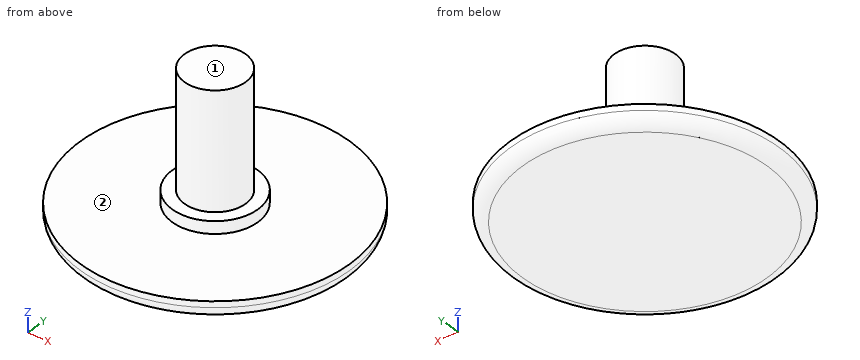
from build123d import *

# Parameters (mm, degrees)
F0_R     = 11
F1_DEPTH = 1.5
F2_R     = 3.5
F3_DEPTH = 1
F4_R     = 2.5
F5_DEPTH = 9.5
F6_R     = 1


with BuildPart() as f1:
    # F0 (on Top) → F1 (new body)
    with BuildSketch(Plane.XY):
        Circle(F0_R)
    extrude(amount=-F1_DEPTH)

    # F2 (on face) → F3 (join)
    with BuildSketch(Plane.XY):
        Circle(F2_R)
    extrude(amount=F3_DEPTH)

    # F4 (on face) → F5 (join)
    with BuildSketch(Plane.XY.offset(1)):
        Circle(F4_R)
    extrude(amount=F5_DEPTH)

    # F6
    f6_edges = [f1.edges().sort_by_distance(p)[0] for p in [
        (-11, 0, -1.5),
    ]]
    fillet(f6_edges, radius=F6_R)


solid = f1.part
Geometry: final body of the model. Coordinates: model frame, mm. Face numbers are marked on the shaded views. A direction names the side the tool comes from. Give positions to 0.01 mm unless a question says otherwise; leave off trailing zeros. Order: outer loops, then holes, each group sorted by start corner. A loop starts at its lowest first (then second) coordinate and runs counter-clockwise, first axis right, second up. Notation, with made-up numbers: (21, 82.25) -> (53, 82.25) arc R27 cw to (53, 117.25) -> close; hole circle Ø2 at (-38, 89). An arc over 180 degrees is marked (long way). Write each question's results on one line, items separated by ' | '.
1) Set-up query: the marked faces 1 and 2. Return all of +Z, -Z, +X, -X, +Y, -Y with unobstructed straight access to the full face (end or side cutting, diameter ignored); none if empty.
Geometry says:
face 1: +Z, +X, -X, +Y, -Y | face 2: +Z
2) Line query: line 1 along Z through (x, y) = (4, 8.5); line 2 along Z through (x, y) = (8, -7.25); line 3 along X through (y, z) = (6, -0.75). Output: solid intervals per line, ascending.
Geometry says:
line 1: z = -1.5 to 0 | line 2: z = -1.1 to 0 | line 3: x = -9.18 to 9.18
3) Cut plane C-C (z = 7.5). Output: boundary loops of the cut face in (x, y), and give its area (3 significant figures).
Geometry says:
outline: circle Ø5 at (0, 0) | area: 19.6 mm²
4) Cut plane A-A (x = 0). Output: boundary loops of the cut face in (y, z).
Geometry says:
outline: (-11, -0.5) arc R1 ccw to (-10, -1.5) -> (10, -1.5) arc R1 ccw to (11, -0.5) -> (11, 0) -> (3.5, 0) -> (3.5, 1) -> (2.5, 1) -> (2.5, 10.5) -> (-2.5, 10.5) -> (-2.5, 1) -> (-3.5, 1) -> (-3.5, 0) -> (-11, 0) -> close
5) First-contact query: pin 1 Ø12 at (x, y) = (-3, 7.5) entering from +Z; pin 2 Ø6 at (x, y) = (6.5, 8) entering from +Z; pin 3 Ø1 at (x, z) = (1, 7.5) entering from -Y. Flat tips, straight axial feed; report the tip coordinate or a pass-through.
Geometry says:
pin 1: stops at z = 10.5 | pin 2: stops at z = 0 | pin 3: stops at y = -2.45
